from build123d import *

# Parameters (mm, degrees)
SKETCH2_W           = 540
SKETCH2_H           = 640
BOSS_EXTRUDE1_DEPTH = 3.175
CUT_EXTRUDE1_DEPTH  = 838.382875765
FILLET1_R           = 10


with BuildPart() as part:
    # Sketch2 → Boss-Extrude1 (new body)
    with BuildSketch(Plane.XY):
        with Locations((270, 320)):
            Rectangle(SKETCH2_W, SKETCH2_H)
    extrude(amount=BOSS_EXTRUDE1_DEPTH)

    # Sketch3 → Cut-Extrude1 (cut, through all)
    with BuildSketch(Plane.XY.offset(3.175)):
        Polygon((0, 640), (0, 560), (80, 640), align=None)
        Polygon((540, 560), (460, 640), (540, 640), align=None)
        Polygon((0, 120), (60, 120), (60, 90), (30, 60), (60, 30), (60, 0), (0, 0), align=None)
        Polygon((540, 0), (540, 120), (480, 120), (480, 90), (510, 60), (480, 30), (480, 0), align=None)
    extrude(amount=-CUT_EXTRUDE1_DEPTH, mode=Mode.SUBTRACT)

    # Fillet1
    fillet1_edges = [part.edges().sort_by_distance(p)[0] for p in [
        (30, 60, 1.5875),
        (510, 60, 1.5875),
    ]]
    fillet(fillet1_edges, radius=FILLET1_R)


solid = part.part
The listing builds one solid part. Answer for the finished solid, in the listing's coordinates (mm). A direction names the side the tool comes from. Coordinates: 2 decimals unless noted, no trailing zeros. Order: outer loops, then holes, each group sorted by start corner. A loop starts at its lowest first (then second) coordinate and runs counter-clockwise, first axis right, second up. Notation, with made-up numbers: M 54.5,-11.75 L 106.5,-11.75 A13 ccw 106.5,10.25 Z; hole C 9,64 d6. An arc over 180 degrees is marked long. Use CSV: the item, a comma, the result in double quotes.
Q1. Section B-B (z = 0.95) is taken. Determine the outline of the cut face in (x, y), then the cut area to 3 significant figures.
Here are the results:
outline,"M 0,120 L 60,120 L 60,90 L 37.07,67.07 A10 ccw 37.07,52.93 L 60,30 L 60,0 L 480,0 L 480,30 L 502.93,52.93 A10 ccw 502.93,67.07 L 480,90 L 480,120 L 540,120 L 540,560 L 460,640 L 80,640 L 0,560 Z"
area,"327,000 mm2"
Q2. A tool of negligible diameter and unlimited length cuts with its end or side. For faces 4 (the flat face through (491, 79, 2)), 5 (the flat face through (39, 599, 2)), from which of +Z, -Z, +X, -X, +Y, -Y can it reach the whole face along a straight path? Write none if from no direction.
Here are the results:
face 4,"+Z, -Z, +X"
face 5,"+Z, -Z, -X, +Y"
Q3. Straight lines are drawn through the part: L1, parallel to X at y = 30.5, z = 0.8; L2, parallel to X at y = 76.5, z = 2.1; L3, parallel to Y at x = 470, z = 2.55. For each, find the intervals that lie inside material, in ascending order.
Here are the results:
L1,"59.5 to 480.5"
L2,"46.5 to 493.5"
L3,"0 to 630"
Q4. Section C-C (y = 575.5) is taken. Determine the outline of the cut face in (x, z) (3 decimals), then the cut area to 3 significant figures.
Here are the results:
outline,"M 15.5,0 L 524.5,0 L 524.5,3.175 L 15.5,3.175 Z"
area,"1,620 mm2"
Q5. Section A-A (x = 50.5) is taken. Determine the outline of the cut face in (y, z) (3 decimals), then the cut area to 3 significant figures.
Here are the results:
outline,"M 39.5,0 L 80.5,0 L 80.5,3.175 L 39.5,3.175 Z; M 120,0 L 610.5,0 L 610.5,3.175 L 120,3.175 Z"
area,"1,690 mm2"
Q6. Determine the mould class of faces 1 (the flat face through (49, 79, 2)), 2 (the flat face through (266, 324, 3.175)), 3 (the flat face through (48, 42, 2)) for opening direction Y: pulls with the +Y half, pulls with the -Y half, needs draft (parallel to the pull), parting line crosses it, or undercut.
Here are the results:
face 1,"undercut"
face 2,"needs draft"
face 3,"pulls with the -Y half"
